The listing builds one solid part. Answer for the finished solid, in the listing's coordinates (mm). Face numbers are marked on the shaded views. A direction names the side the tool comes from. Coordinates: 2 decimals unless noted, no trailing zeros. Loops run counter-clockwise (first coordinate to the right, second up) from the corner with the lowest first, then second, coordinate; pieces in that order, holes last. Notation, with made-up numbers: (-25, 40) - (7, 40) arc R11 cw to (7, 59) - close; hole circle Ø10 at (20, 49.5). An arc over 180 degrees is marked (long way). Return JSON: item names as keys, results as strings. Group by question number.
1. Which of the six approach directions +Z, -Z, +X, -X, +Y, -Y give full straight-line access (tool end or side, diameter ignored) to the marked faces 1, 2, 3, 4 and 5?
2. Section A-A (x = 10.25) is taken. Write down the section's boundary in (y, z), and give its area (3 significant figures).
3. Find the intervals of material crossed by line 1 along Z through (x, y) = (11.5, 0); line 2 along Y through (x, z) = (5.5, 0), in increasing order.
4. The mould has two halves that part along Z. Classify the marked faces 6, 7 and 8: pulls with the +Z half, pulls with the -Z half, needs draft (parallel to the pull), parting line crosses it, or undercut.
5. Section B-B (x = 5.75) is taken. Write down the section's boundary in (y, z), and give its area (3 significant figures).
6. Each of these flat-tipped pins is pushed along its axis until it touches: P1, Ø3, axis at y = -13.5, z = 11.5, coming from the +X side; P2, Ø5, axis at x = 9.5, y = 8.5, coming from the -Z side; P3, Ø2, axis at y = -11.5, z = 8, coming from the -X side. Where does it stop, or does it pass through?
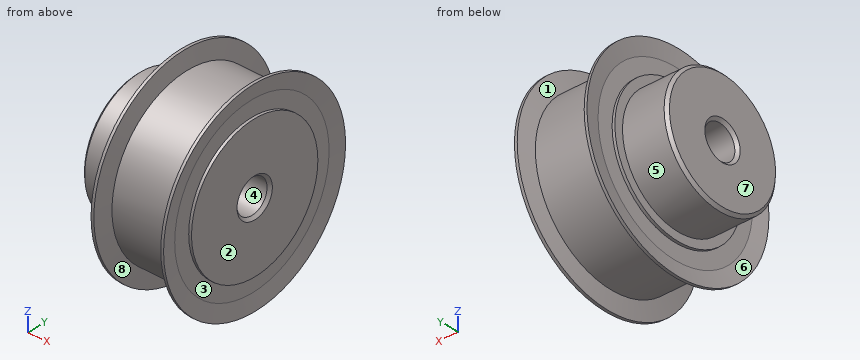
```python
from build123d import *

# Parameters (mm, degrees)
FASE1_SIZE = 0.5


with BuildPart() as part:
    # Layout → Rotation1 (revolve)
    with BuildSketch(Plane.XY):
        Polygon((0, 3), (0, 11), (7.962375299, 11), (7.962375299, 12.5), (8.462375299, 12.5), (8.462375299, 15.271049232), (7.981187649, 18), (8.481187649, 18), (9.010168592, 15), (19.952206707, 15), (20.481187649, 18), (20.981187649, 18), (20.5, 15.271049232), (20.5, 12.5), (21, 12.5), (21, 3), align=None)
    revolve(axis=Axis((21, 0, 0), (-1, 0, 0)))

    # Fase1
    fase1_edges = [part.edges().sort_by_distance(p)[0] for p in [
        (0, -11, 0),
        (0, -3, 0),
        (21, -3, 0),
    ]]
    chamfer(fase1_edges, length=FASE1_SIZE)


solid = part.part
```
The answers:
{
 "1": {"face 1": "none", "face 2": "+Z, -Z, +X, +Y, -Y", "face 3": "+X", "face 4": "+X, -X", "face 5": "-X"},
 "2": {"outline": "circle Ø30 at (0, 0); hole circle Ø6 at (0, 0)", "area": "679 mm2"},
 "3": {"line 1": "z = -15 to -3, 3 to 15", "line 2": "y = -11 to -3, 3 to 11"},
 "4": {"face 6": "undercut", "face 7": "needs draft", "face 8": "parting line crosses it"},
 "5": {"outline": "circle Ø22 at (0, 0); hole circle Ø6 at (0, 0)", "area": "352 mm2"},
 "6": {"P1": "stops at x = 20.98", "P2": "stops at z = -16.89", "P3": "stops at x = 8.46"}
}
